```python
from build123d import *

# Parameters (mm, degrees)
F1_DEPTH = 3
F2_DEPTH = 25
F3_DEPTH = 25


with BuildPart() as f1:
    # F0 (on Top) → F1 (new body)
    with BuildSketch(Plane.XY):
        with BuildLine():
            Line((-480.661231, 172.248819), (-755.661231, 172.248819))
            Line((-755.661231, 172.248819), (-755.661231, -64.751181))
            Line((-755.661231, -64.751181), (-555.661231, -64.751181))
            Line((-555.661231, -64.751181), (-555.661231, -264.751181))
            Line((-555.661231, -264.751181), (-380.661231, -264.751181))
            ThreePointArc((-380.661231, -264.751181), (-350.661231, -234.751181), (-320.661231, -264.751181))
            Line((-320.661231, -264.751181), (534.338769, -264.751181))
            Line((534.338769, -264.751181), (534.338769, -64.751181))
            Line((534.338769, -64.751181), (734.338769, -64.751181))
            Line((734.338769, -64.751181), (734.338769, 172.248819))
            Line((734.338769, 172.248819), (25.338769, 172.248819))
            Line((25.338769, 172.248819), (-38.161231, 172.248819))
            Line((-38.161231, 172.248819), (-402.510524, 172.248819))
            Line((-402.510524, 172.248819), (-417.161231, 172.248819))
            Line((-417.161231, 172.248819), (-480.661231, 172.248819))
        make_face()
        with BuildLine():
            ThreePointArc((-480.161231, 171.248819), (-481.014785, 170.895266), (-480.661231, 171.748819))
            ThreePointArc((-480.661231, 171.748819), (-480.307678, 171.602373), (-480.161231, 171.248819))
        make_face(mode=Mode.SUBTRACT)
        with BuildLine():
            ThreePointArc((-417.161231, 170.748819), (-417.661231, 171.248819), (-417.161231, 171.748819))
            ThreePointArc((-417.161231, 171.748819), (-416.807678, 171.602373), (-416.661231, 171.248819))
            ThreePointArc((-416.661231, 171.248819), (-416.807678, 170.895266), (-417.161231, 170.748819))
        make_face(mode=Mode.SUBTRACT)
        with BuildLine():
            ThreePointArc((-38.161231, 170.748819), (-38.661231, 171.248819), (-38.161231, 171.748819))
            ThreePointArc((-38.161231, 171.748819), (-37.807678, 171.602373), (-37.661231, 171.248819))
            ThreePointArc((-37.661231, 171.248819), (-37.807678, 170.895266), (-38.161231, 170.748819))
        make_face(mode=Mode.SUBTRACT)
        with BuildLine():
            ThreePointArc((25.338769, 170.748819), (24.838769, 171.248819), (25.338769, 171.748819))
            ThreePointArc((25.338769, 171.748819), (25.692322, 171.602373), (25.838769, 171.248819))
            ThreePointArc((25.838769, 171.248819), (25.692322, 170.895266), (25.338769, 170.748819))
        make_face(mode=Mode.SUBTRACT)
    extrude(amount=F1_DEPTH)

    # F0 (on Top) → F2 (cut)
    with BuildSketch(Plane.XY):
        with BuildLine():
            ThreePointArc((-480.161231, 171.248819), (-480.307678, 171.602373), (-480.661231, 171.748819))
            ThreePointArc((-480.661231, 171.748819), (-481.014785, 170.895266), (-480.161231, 171.248819))
        make_face()
        with BuildLine():
            Line((-480.661231, 172.248819), (-755.661231, 172.248819))
            Line((-755.661231, 172.248819), (-755.661231, -64.751181))
            Line((-755.661231, -64.751181), (-555.661231, -64.751181))
            Line((-555.661231, -64.751181), (-555.661231, -264.751181))
            Line((-555.661231, -264.751181), (-380.661231, -264.751181))
            ThreePointArc((-380.661231, -264.751181), (-350.661231, -234.751181), (-320.661231, -264.751181))
            Line((-320.661231, -264.751181), (534.338769, -264.751181))
            Line((534.338769, -264.751181), (534.338769, -64.751181))
            Line((534.338769, -64.751181), (734.338769, -64.751181))
            Line((734.338769, -64.751181), (734.338769, 172.248819))
            Line((734.338769, 172.248819), (25.338769, 172.248819))
            Line((25.338769, 172.248819), (-38.161231, 172.248819))
            Line((-38.161231, 172.248819), (-402.510524, 172.248819))
            Line((-402.510524, 172.248819), (-417.161231, 172.248819))
            Line((-417.161231, 172.248819), (-480.661231, 172.248819))
        make_face()
        with BuildLine():
            ThreePointArc((-480.161231, 171.248819), (-481.014785, 170.895266), (-480.661231, 171.748819))
            ThreePointArc((-480.661231, 171.748819), (-480.307678, 171.602373), (-480.161231, 171.248819))
        make_face(mode=Mode.SUBTRACT)
        with BuildLine():
            ThreePointArc((-417.161231, 170.748819), (-417.661231, 171.248819), (-417.161231, 171.748819))
            ThreePointArc((-417.161231, 171.748819), (-416.807678, 171.602373), (-416.661231, 171.248819))
            ThreePointArc((-416.661231, 171.248819), (-416.807678, 170.895266), (-417.161231, 170.748819))
        make_face(mode=Mode.SUBTRACT)
        with BuildLine():
            ThreePointArc((-38.161231, 170.748819), (-38.661231, 171.248819), (-38.161231, 171.748819))
            ThreePointArc((-38.161231, 171.748819), (-37.807678, 171.602373), (-37.661231, 171.248819))
            ThreePointArc((-37.661231, 171.248819), (-37.807678, 170.895266), (-38.161231, 170.748819))
        make_face(mode=Mode.SUBTRACT)
        with BuildLine():
            ThreePointArc((25.338769, 170.748819), (24.838769, 171.248819), (25.338769, 171.748819))
            ThreePointArc((25.338769, 171.748819), (25.692322, 171.602373), (25.838769, 171.248819))
            ThreePointArc((25.838769, 171.248819), (25.692322, 170.895266), (25.338769, 170.748819))
        make_face(mode=Mode.SUBTRACT)
        with BuildLine():
            ThreePointArc((-320.661231, -264.751181), (-350.661231, -234.751181), (-380.661231, -264.751181))
            Line((-380.661231, -264.751181), (-320.661231, -264.751181))
        make_face()
    extrude(amount=-F2_DEPTH, mode=Mode.SUBTRACT)

    # F0 (on Top) → F3 (cut)
    with BuildSketch(Plane.XY):
        with BuildLine():
            ThreePointArc((-480.161231, 171.248819), (-480.307678, 171.602373), (-480.661231, 171.748819))
            ThreePointArc((-480.661231, 171.748819), (-481.014785, 170.895266), (-480.161231, 171.248819))
        make_face()
        with BuildLine():
            Line((-480.661231, 172.248819), (-755.661231, 172.248819))
            Line((-755.661231, 172.248819), (-755.661231, -64.751181))
            Line((-755.661231, -64.751181), (-555.661231, -64.751181))
            Line((-555.661231, -64.751181), (-555.661231, -264.751181))
            Line((-555.661231, -264.751181), (-380.661231, -264.751181))
            ThreePointArc((-380.661231, -264.751181), (-350.661231, -234.751181), (-320.661231, -264.751181))
            Line((-320.661231, -264.751181), (534.338769, -264.751181))
            Line((534.338769, -264.751181), (534.338769, -64.751181))
            Line((534.338769, -64.751181), (734.338769, -64.751181))
            Line((734.338769, -64.751181), (734.338769, 172.248819))
            Line((734.338769, 172.248819), (25.338769, 172.248819))
            Line((25.338769, 172.248819), (-38.161231, 172.248819))
            Line((-38.161231, 172.248819), (-402.510524, 172.248819))
            Line((-402.510524, 172.248819), (-417.161231, 172.248819))
            Line((-417.161231, 172.248819), (-480.661231, 172.248819))
        make_face()
        with BuildLine():
            ThreePointArc((-480.161231, 171.248819), (-481.014785, 170.895266), (-480.661231, 171.748819))
            ThreePointArc((-480.661231, 171.748819), (-480.307678, 171.602373), (-480.161231, 171.248819))
        make_face(mode=Mode.SUBTRACT)
        with BuildLine():
            ThreePointArc((-417.161231, 170.748819), (-417.661231, 171.248819), (-417.161231, 171.748819))
            ThreePointArc((-417.161231, 171.748819), (-416.807678, 171.602373), (-416.661231, 171.248819))
            ThreePointArc((-416.661231, 171.248819), (-416.807678, 170.895266), (-417.161231, 170.748819))
        make_face(mode=Mode.SUBTRACT)
        with BuildLine():
            ThreePointArc((-38.161231, 170.748819), (-38.661231, 171.248819), (-38.161231, 171.748819))
            ThreePointArc((-38.161231, 171.748819), (-37.807678, 171.602373), (-37.661231, 171.248819))
            ThreePointArc((-37.661231, 171.248819), (-37.807678, 170.895266), (-38.161231, 170.748819))
        make_face(mode=Mode.SUBTRACT)
        with BuildLine():
            ThreePointArc((25.338769, 170.748819), (24.838769, 171.248819), (25.338769, 171.748819))
            ThreePointArc((25.338769, 171.748819), (25.692322, 171.602373), (25.838769, 171.248819))
            ThreePointArc((25.838769, 171.248819), (25.692322, 170.895266), (25.338769, 170.748819))
        make_face(mode=Mode.SUBTRACT)
        with BuildLine():
            ThreePointArc((-320.661231, -264.751181), (-350.661231, -234.751181), (-380.661231, -264.751181))
            Line((-380.661231, -264.751181), (-320.661231, -264.751181))
        make_face()
    extrude(amount=-F3_DEPTH, mode=Mode.SUBTRACT)


solid = f1.part
```
Can you work these out from the model? Positions are in its coordinate system, mm. Coordinates: 2 decimals unless noted, no trailing zeros. Loops run counter-clockwise (first coordinate to the right, second up) from the corner with the lowest first, then second, coordinate; pieces in that order, holes last. Notation, with made-up numbers: M 28,12.25 L 54,12.25 A18 cw 54,31.25 Z; hole C -27.75,61 d2. An arc over 180 degrees is marked long. Put each result on its own line as item: value. Start each with the question number.
(1) I need wall thicknesses on probe 1 along X at (y, z) = (-237.5, 0.3); probe 2 along X at (y, z) = (-144, 2); probe 3 along Y at (x, z) = (554, 2.8). Which ranges of each line are inside material? Lowest first, please.
(2) Imagine slicing it at B-B on x = 625. List the corners of the cut face in (y, z) for me, and give its area (3 significant figures).
(3) Will these pins go through, and if not, where does the flat tip stop? pin 1 Ø1.5 at (x, z) = (646, 1.5) entering from -Y; pin 2 Ø0.9 at (x, y) = (-480.66, 171.25) entering from -Z.
(4) Imagine slicing it at A-A on z = 1.2. List the corners of the cut face in (x, y) for me, and give its area (3 significant figures).
(5) Imagine slicing it at C-C on y = -89.5. List the corners of the cut face in (x, z) for me.
Worked answers:
1. probe 1: x = -555.66 to -363.21, -338.12 to 534.34
1. probe 2: x = -555.66 to 534.34
1. probe 3: y = -64.75 to 172.25
2. outline: M -64.75,0 L 172.25,0 L 172.25,3 L -64.75,3 Z
2. area: 711 mm2
3. pin 1: stops at y = -64.75
3. pin 2: passes through
4. outline: M -755.66,-64.75 L -555.66,-64.75 L -555.66,-264.75 L -380.66,-264.75 A30 cw -320.66,-264.75 L 534.34,-264.75 L 534.34,-64.75 L 734.34,-64.75 L 734.34,172.25 L -755.66,172.25 Z; hole C -480.66,171.25 d1; hole M -417.16,170.75 A0.5 ccw -416.66,171.25 A0.5 ccw long Z; hole M -38.16,170.75 A0.5 ccw -37.66,171.25 A0.5 ccw long Z; hole M 25.34,170.75 A0.5 ccw 25.84,171.25 A0.5 ccw long Z
4. area: 570,000 mm2
5. outline: M -555.66,0 L 534.34,0 L 534.34,3 L -555.66,3 Z
